from build123d import *

# Parameters (mm, degrees)
F0_R      = 25.4
F1_DEPTH  = 6.35
F2_R      = 22.225
F3_DEPTH  = 12.7
F4_R      = 25.4
F5_DEPTH  = 6.35
F7_D      = 6.35
F7_DEPTH  = 3.175
F7_TIP    = 1.9077324654
F8_R      = 1.6002
F9_R      = 6.35
F10_DEPTH = 25.401


with BuildPart() as f1:
    # F0 (on Front) → F1 (new body)
    with BuildSketch(Plane.XZ):
        Circle(F0_R)
    extrude(amount=F1_DEPTH)

    # F2 (on face) → F3 (join)
    with BuildSketch(Plane.XZ.offset(6.35)):
        Circle(F2_R)
    extrude(amount=F3_DEPTH)

    # F4 (on face) → F5 (join)
    with BuildSketch(Plane.XZ.offset(19.05)):
        Circle(F4_R)
    extrude(amount=F5_DEPTH)

    # F7
    with Locations(Plane.XZ.offset(25.4)):
        with Locations((0, 19.05), (19.05, 0), (0, -19.05), (-19.05, 0)):
            Hole(F7_D / 2, depth=F7_DEPTH)
            with Locations((0, 0, -(F7_DEPTH + F7_TIP / 2))):  # 118° drill point
                Cone(0, F7_D / 2, F7_TIP, mode=Mode.SUBTRACT)

    # F8
    f8_edges = [f1.edges().sort_by_distance(p)[0] for p in [
        (-25.4, -25.4, 0),
        (-25.4, -19.05, 0),
        (-25.4, -6.35, 0),
        (-25.4, 0, 0),
    ]]
    fillet(f8_edges, radius=F8_R)

    # F9 (on face) → F10 (cut, through all)
    with BuildSketch(Plane.XZ.offset(25.4)):
        Circle(F9_R)
    extrude(amount=-F10_DEPTH, mode=Mode.SUBTRACT)


solid = f1.part
The model under review builds one solid part; all positions refer to its coordinate system, in mm. A direction names the side the tool comes from. Coordinates: 2 decimals unless noted, no trailing zeros. Write each loop counter-clockwise with the first axis right and the second up, starting at its lowest first coordinate (ties: lowest second). Pieces come first, ordered by that corner, then holes. Notation, with made-up numbers: M 20.5,4.25 L 25.5,4.25 A29 cw 25.5,40.25 Z; hole C -24,-20 d7. An arc over 180 degrees is marked long. Put each result on its own line as item: value.
1) Wall thickness on probe 1 along Z at (x, y) = (0, -23.05) (3 decimals); probe 2 along Y at (x, z) = (14, 19.5); probe 3 along Z at (x, y) = (0, -16) (3 decimals): over which ranges is each line inside the solid? List them lowest first. Write a range as [from, to].
Computed:
probe 1: z = [-25.4, -22.225], [-15.875, -6.35], [6.35, 15.875], [22.225, 25.4]
probe 2: y = [-25.39, -19.06], [-6.34, -0.01]
probe 3: z = [-22.225, -6.35], [6.35, 22.225]
2) Clearance check with flat-ended pins moving along their axes: pin 1 Ø4 at (x, y) = (20, -21) entering from -Z; pin 2 Ø1.5 at (x, y) = (4, -5.5) entering from +Z; pin 3 Ø10 at (y, z) = (-3.5, 12) entering from -X. State where each tip first meets the part, or that it passes through.
Computed:
pin 1: stops at z = -17.92
pin 2: stops at z = 25.15
pin 3: stops at x = -24.42
3) Add section A-A on y = -12. Give the boundary of the cut face in (x, z) (3 decimals).
Computed:
outline: C 0,0 d44.45; hole C 0,0 d12.7
4) For faces 1 (the flat face through (-20, -19.05, 11)), 2 (the cylindrical face through (16.02, -23.79, 0.95)), 3 (the flat face through (5, -25.4, -5)), list the 3-axis set-ups (+Z, -Z, +X, -X, +Y, -Y) from which the entire face can be reached by the end or side of a thin tool; tool diameter is ignored.
Computed:
face 1: none
face 2: -Y
face 3: +Z, -Z, +X, -X, -Y
5) Draft analysis for pull direction Y (two halves, no side actions). For faces 4 (the conical face through (-0.12, -20.65, 18.51)), 5 (the flat face through (5, 0, -5)), 6 (the flat face through (-20, -6.35, 11)), 7 (the cylindrical face through (0.69, -23.79, 15.95)), state which applies: released by +Y, released by -Y, zero draft, split by the parting line, or undercut.
Computed:
face 4: released by -Y
face 5: released by +Y
face 6: undercut
face 7: zero draft
